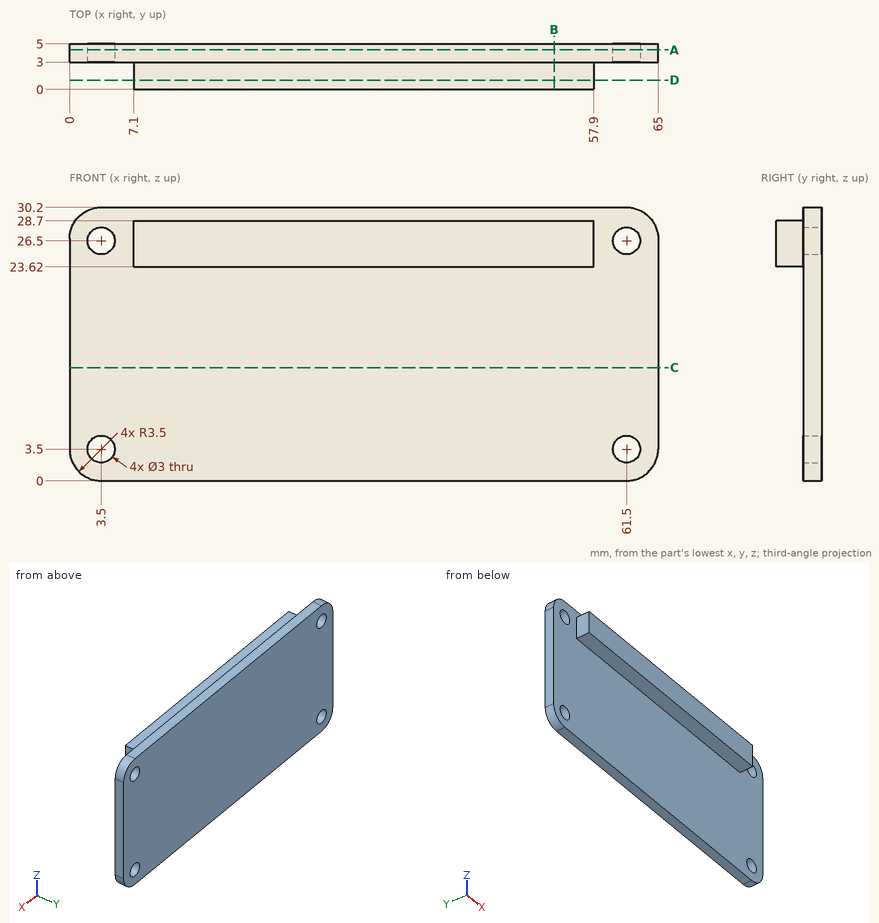
Design review of the part shown in the three views and the two pictorial views. Dimensions are in mm from the part's minimum x, y and z. Round coordinates to 2 decimals unless told otherwise and drop trailing zeros. Write each loop counter-clockwise with the first axis right and the second up, starting at its lowest first coordinate (ties: lowest second). Pieces come first, ordered by that corner, then holes. Notation, with made-up numbers: (63.5, -26.5) - (107.5, -26.5) arc R7 ccw to (107.5, -21.5) - close; hole circle Ø10 at (-19.5, 6.5). An arc over 180 degrees is marked (long way). Return JSON: item names as keys, results as strings. Group by question number.
Item 1: We need section B-B on x = 53.5. Write out the cut boundary in (y, z).
Item 2: Insertion check: P1, Ø0.9, axis at x = 27, y = 1.5, coming from the +Z side; P2, Ø2.5, axis at x = 3.5, z = 26.5, coming from the -Y side; P3, Ø5, axis at x = 17.5, z = 20.5, coming from the -Y side; P4, Ø0.9, axis at y = 2, z = 26, coming from the -X side. Each pin has a flat end and moves straight along its axis. Give the tip position at first contact, or say it passes through.
Item 3: We need section A-A on y = 4.35. Write out the cut boundary in (x, z), and give its area (3 significant figures).
Item 4: We need section D-D on y = 1. Write out the cut boundary in (x, z).
Item 5: For probe 1 along Z at (x, y) = (61.5, 4.15); probe 2 along X at (y, z) = (3.8, 26.5); probe 3 along X at (y, z) = (3.5, 27), list the stretches that pass through material, from the lowest coordinate up. Write a range as [from, to].
Item 6: We need section C-C on z = 12.5. Write out the cut boundary in (x, y), and give its area (3 significant figures).
Model answer:
{
 "1": {"outline": "(0, 23.62) - (3, 23.62) - (3, 0) - (5, 0) - (5, 30.2) - (3, 30.2) - (3, 28.7) - (0, 28.7) - close"},
 "2": {"P1": "stops at z = 28.7", "P2": "passes through", "P3": "stops at y = 3", "P4": "stops at x = 7.1"},
 "3": {"outline": "(0, 3.5) arc R3.5 ccw to (3.5, 0) - (61.5, 0) arc R3.5 ccw to (65, 3.5) - (65, 26.7) arc R3.5 ccw to (61.5, 30.2) - (3.5, 30.2) arc R3.5 ccw to (0, 26.7) - close; hole circle Ø3 at (3.5, 3.5); hole circle Ø3 at (3.5, 26.5); hole circle Ø3 at (61.5, 3.5); hole circle Ø3 at (61.5, 26.5)", "area": "1,920 mm²"},
 "4": {"outline": "(7.1, 23.62) - (57.9, 23.62) - (57.9, 28.7) - (7.1, 28.7) - close"},
 "5": {"probe 1": "z = [0, 2], [5, 25], [28, 30.2]", "probe 2": "x = [0, 2], [5, 60], [63, 65]", "probe 3": "x = [0.01, 2.09], [4.91, 60.09], [62.91, 64.99]"},
 "6": {"outline": "(0, 3) - (65, 3) - (65, 5) - (0, 5) - close", "area": "130 mm²"}
}
